Here's how the part is built. I have some questions about the finished solid (model axes, mm). A direction names the side the tool comes from. Give positions to 0.01 mm unless a question says otherwise; leave off trailing zeros. Loops run counter-clockwise (first coordinate to the right, second up) from the corner with the lowest first, then second, coordinate; pieces in that order, holes last. Notation, with made-up numbers: (-24.75, 35.25) -> (-4.75, 35.25) arc R29 cw to (-4.75, 63.25) -> close; hole circle Ø3 at (3, 39). An arc over 180 degrees is marked (long way). Answer in a Markdown table with one row per item. Add a question column.
Item 1: If I drill on line 1 (X direction, y = -2.5, z = -19.5); line 2 (Z direction, x = -12.5, y = -3.25); line 3 (Z direction, x = -12, y = -0.5), over which ranges is the centre line in solid material (lowest first)?
Item 2: For P1, Ø22.5, axis at x = -11.41, z = -11.41, coming from the -Y side; P2, Ø7, axis at x = 0, z = 0, coming from the +Y side; P3, Ø12, axis at x = 11, z = -3, coming from the +Y side, each with a flat end and sliding along its axis, tell me the tip position at first contact or that it passes through.
Item 3: If we section it at A-A (z = 10.5): Write out the boundary of the cut face in (x, y).
Item 4: If we section it at C-C (x = 19): Write out the boundary of the cut face in (y, z), then the cut area to 3 significant figures.
Item 5: If we section it at D-D (z = -1): Write out the boundary of the cut face in (x, y).
Item 6: Which directions (+Z, -Z, +X, -X, +Y, -Y) give clear straight access to the entire face, cutting with the end or side of a thin tool? Please do faces 4 (the face through (4.42, -1.97, -4.45)), 5 (the face through (-0.59, -0.99, 4.46)).
Item 7: We'd pull the mould along Z, two halves only. Please class faces 1 (the face through (-3.06, -1.97, -12.7)), 2 (the face through (-0.59, -5.97, 4.46)), 3 (the face through (2, 0, 4.4)): released by +Z, released by -Z, zero draft, split by the parting line, or undercut.
Item 8: If we section it at B-B (y = -2.75): Give the number of separate pieces and of enclosed holes in the cut face, then the cut area to 3 significant figures.
```python
from build123d import *

# Parameters (mm, degrees)
F0_R     = 4.5
F1_DEPTH = 8
F0_R_2   = 29
F0_R_3   = 27
F2_DEPTH = 4
F3_DEPTH = 2


with BuildPart() as f1:
    # F0 (on Front) → F1 (new body)
    with BuildSketch(Plane.XZ):
        Circle(F0_R)
    extrude(amount=F1_DEPTH)

    # F0 (on Front) → F2 (join)
    with BuildSketch(Plane.XZ):
        Circle(F0_R_2)
        Circle(F0_R_3, mode=Mode.SUBTRACT)
        Circle(F0_R_3)
        with BuildLine():
            ThreePointArc((4.3516162867, -22.646052221), (-0.1431680004, -25.9977219705), (-4.4156935051, -22.3669780097))
            Line((-4.4156935051, -22.3669780097), (0, -7.75))
            Line((0, -7.75), (4.3516162867, -22.646052221))
        make_face(mode=Mode.SUBTRACT)
        with BuildLine():
            ThreePointArc((-3.8942970998, -17.7984822768), (-18.3847763109, -18.3847763109), (-17.7984822768, -3.8942970998))
            Line((-17.7984822768, -3.8942970998), (-7.75, -2.25))
            ThreePointArc((-7.75, -2.25), (-4.4349924254, -4.4349924254), (-2.25, -7.75))
            Line((-2.25, -7.75), (-3.8942970998, -17.7984822768))
        make_face(mode=Mode.SUBTRACT)
        with BuildLine():
            Line((3.9160785154, -17.9315909272), (2.241457342, -7.6977948676))
            ThreePointArc((2.241457342, -7.6977948676), (4.4638924206, -4.4067558), (7.8040467228, -2.2588440092))
            Line((7.8040467228, -2.2588440092), (17.6630391225, -3.8721336746))
            ThreePointArc((17.6630391225, -3.8721336746), (18.4127954662, -18.3556588455), (3.9160785154, -17.9315909272))
        make_face(mode=Mode.SUBTRACT)
        with BuildLine():
            ThreePointArc((-22.3669780097, -4.4156935051), (-26, 0), (-22.3669780097, 4.4156935051))
            Line((-22.3669780097, 4.4156935051), (-7.75, 0))
            Line((-7.75, 0), (-22.3669780097, -4.4156935051))
        make_face(mode=Mode.SUBTRACT)
        with BuildLine():
            Line((-7.75, 2.25), (-17.7984822768, 3.8942970998))
            ThreePointArc((-17.7984822768, 3.8942970998), (-18.3847763109, 18.3847763109), (-3.8942970998, 17.7984822768))
            Line((-3.8942970998, 17.7984822768), (-2.25, 7.75))
            ThreePointArc((-2.25, 7.75), (-4.4349924254, 4.4349924254), (-7.75, 2.25))
        make_face(mode=Mode.SUBTRACT)
        Circle(F0_R, mode=Mode.SUBTRACT)
        with BuildLine():
            Line((17.7984822768, 3.8942970998), (7.75, 2.25))
            ThreePointArc((7.75, 2.25), (4.4349924254, 4.4349924254), (2.25, 7.75))
            Line((2.25, 7.75), (3.8942970998, 17.7984822768))
            ThreePointArc((3.8942970998, 17.7984822768), (18.3847763109, 18.3847763109), (17.7984822768, 3.8942970998))
        make_face(mode=Mode.SUBTRACT)
        with BuildLine():
            ThreePointArc((22.3669780097, 4.4156935051), (26, 0), (22.3669780097, -4.4156935051))
            Line((22.3669780097, -4.4156935051), (7.75, 0))
            Line((7.75, 0), (14.262410288, 1.9673565762))
            Line((14.262410288, 1.9673565762), (22.3669780097, 4.4156935051))
        make_face(mode=Mode.SUBTRACT)
        with BuildLine():
            ThreePointArc((-4.4156935051, 22.3669780097), (0, 26), (4.4156935051, 22.3669780097))
            Line((4.4156935051, 22.3669780097), (0, 7.75))
            Line((0, 7.75), (-4.4156935051, 22.3669780097))
        make_face(mode=Mode.SUBTRACT)
    extrude(amount=F2_DEPTH)

    # F0 (on Front) → F3 (cut)
    with BuildSketch(Plane.XZ):
        Circle(F0_R)
    extrude(amount=F3_DEPTH, mode=Mode.SUBTRACT)


solid = f1.part
```
Recorded:
| question | item | result |
|---|---|---|
| 1 | line 1 | x = -21.47 to -17.05, -5.77 to -3.55, 3.43 to 5.65, 17.07 to 21.47 |
| 1 | line 2 | z = -26.17 to -21.21, -3.03 to -1.43, 1.43 to 3.03, 21.21 to 26.17 |
| 1 | line 3 | z = -26.4 to -21.26, -2.95 to -1.28, 1.28 to 2.95, 21.26 to 26.4 |
| 2 | P1 | stops at y = -4 |
| 2 | P2 | stops at y = -2 |
| 2 | P3 | stops at y = 0 |
| 3 | outline | (-27.03, -4) -> (-21.23, -4) -> (-21.23, 0) -> (-27.03, 0) -> close; (-2.7, -4) -> (-0.83, -4) -> (-0.83, 0) -> (-2.7, 0) -> close; (0.83, -4) -> (2.7, -4) -> (2.7, 0) -> (0.83, 0) -> close; (21.23, -4) -> (27.03, -4) -> (27.03, 0) -> (21.23, 0) -> close |
| 4 | outline | (-4, -21.91) -> (0, -21.91) -> (0, -17.7) -> (-4, -17.7) -> close; (-4, -5.22) -> (0, -5.22) -> (0, -3.4) -> (-4, -3.4) -> close; (-4, 3.4) -> (0, 3.4) -> (0, 5.11) -> (-4, 5.11) -> close; (-4, 17.71) -> (0, 17.71) -> (0, 21.91) -> (-4, 21.91) -> close |
| 4 | area | 47.8 mm^2 |
| 5 | outline | (-28.98, -4) -> (-25.89, -4) -> (-25.89, 0) -> (-28.98, 0) -> close; (-11.06, -4) -> (-4.39, -4) -> (-4.39, -8) -> (4.39, -8) -> (4.39, -4) -> (11.06, -4) -> (11.06, 0) -> (4.39, 0) -> (4.39, -2) -> (-4.39, -2) -> (-4.39, 0) -> (-11.06, 0) -> close; (25.89, -4) -> (28.98, -4) -> (28.98, 0) -> (25.89, 0) -> close |
| 6 | face 4 | +Y, -Y |
| 6 | face 5 | +Y |
| 7 | face 1 | undercut |
| 7 | face 2 | split by the parting line |
| 7 | face 3 | zero draft |
| 8 | separate pieces | 1 |
| 8 | enclosed holes | 8 |
| 8 | area | 1,140 mm^2 |
